```python
from build123d import *

# Parameters (mm, degrees)
SKETCH2_W            = 40
SKETCH2_H            = 40
SKETCH2_R            = 2.5
SKETCH2_R_2          = 16
SKETCH2_R_3          = 6.5
SKETCH2_R_4          = 12
BOSS_EXTRUDE5_DEPTH  = 2.5
BOSS_EXTRUDE8_START  = 2.5
SKETCH2_9_R          = 16
SKETCH2_9_R_2        = 6.5
SKETCH2_9_R_3        = 12
BOSS_EXTRUDE8_DEPTH  = 6
BOSS_EXTRUDE10_START = -32.5
SKETCH2_12_R         = 12
SKETCH2_12_R_2       = 6.5
BOSS_EXTRUDE10_DEPTH = 30
FILLET1_R            = 3
FILLET2_R            = 0.5
FILLET3_R            = 5
FILLET4_R            = 1


with BuildPart() as part:
    # Sketch2 → Boss-Extrude5 (new, symmetric)
    # profile 1 of 3: a face of its own
    with BuildSketch(Plane.XY):
        Rectangle(SKETCH2_W, SKETCH2_H)
        with Locations((-15, -15)):
            Circle(SKETCH2_R, mode=Mode.SUBTRACT)
        with Locations((15, -15)):
            Circle(SKETCH2_R, mode=Mode.SUBTRACT)
        with Locations((15, 15)):
            Circle(SKETCH2_R, mode=Mode.SUBTRACT)
        with Locations((-15, 15)):
            Circle(SKETCH2_R, mode=Mode.SUBTRACT)
        Circle(SKETCH2_R_2, mode=Mode.SUBTRACT)
    # profile 2 of 3: a face of its own
    with BuildSketch(Plane.XY):
        Circle(SKETCH2_R_2)
        Circle(SKETCH2_R_3, mode=Mode.SUBTRACT)
    # profile 3 of 3: a face of its own
    with BuildSketch(Plane.XY):
        Circle(SKETCH2_R_4)
        Circle(SKETCH2_R_3, mode=Mode.SUBTRACT)
    extrude(amount=BOSS_EXTRUDE5_DEPTH, both=True)

    # Sketch2<9> → Boss-Extrude8 (add)
    # profile 1 of 2: a face of its own
    with BuildSketch(Plane.XY.offset(BOSS_EXTRUDE8_START)):
        Circle(SKETCH2_9_R)
        Circle(SKETCH2_9_R_2, mode=Mode.SUBTRACT)
    # profile 2 of 2: a face of its own
    with BuildSketch(Plane.XY.offset(BOSS_EXTRUDE8_START)):
        Circle(SKETCH2_9_R_3)
        Circle(SKETCH2_9_R_2, mode=Mode.SUBTRACT)
    extrude(amount=BOSS_EXTRUDE8_DEPTH)

    # Sketch2<12> → Boss-Extrude10 (add)
    with BuildSketch(Plane.XY.offset(BOSS_EXTRUDE10_START)):
        Circle(SKETCH2_12_R)
        Circle(SKETCH2_12_R_2, mode=Mode.SUBTRACT)
    extrude(amount=BOSS_EXTRUDE10_DEPTH)

    # Fillet1
    fillet1_edges = [part.edges().sort_by_distance(p)[0] for p in [
        (20, -20, 0),
        (-20, -20, 0),
        (-20, 20, 0),
        (20, 20, 0),
    ]]
    fillet(fillet1_edges, radius=FILLET1_R)

    # Fillet2
    fillet2_edges = [part.edges().sort_by_distance(p)[0] for p in [
        (0, 20, -2.5),
        (20, 0, -2.5),
        (0, -20, -2.5),
        (-20, 0, -2.5),
        (-19.121320344, 19.121320344, -2.5),
        (-19.121320344, -19.121320344, -2.5),
        (19.121320344, -19.121320344, -2.5),
        (19.121320344, 19.121320344, -2.5),
    ]]
    fillet(fillet2_edges, radius=FILLET2_R)

    # Fillet3
    fillet3_edges = [part.edges().sort_by_distance(p)[0] for p in [
        (-12, 0, -2.5),
    ]]
    fillet(fillet3_edges, radius=FILLET3_R)

    # Fillet4
    fillet4_edges = [part.edges().sort_by_distance(p)[0] for p in [
        (-12, 0, -32.5),
    ]]
    fillet(fillet4_edges, radius=FILLET4_R)


solid = part.part
```
Geometry: final body of the model. Coordinates: model frame, mm. A direction names the side the tool comes from. Coordinates: 2 decimals unless noted, no trailing zeros. Order: outer loops, then holes, each group sorted by start corner. A loop starts at its lowest first (then second) coordinate and runs counter-clockwise, first axis right, second up. Notation, with made-up numbers: (9, -15) - (64, -15) arc R25 cw to (64, 18) - close; hole circle Ø10 at (72.25, 68). An arc over 180 degrees is marked (long way). Return JSON: item names as keys, results as strings. Group by question number.
1. Pin query (flat end, axial travel): pin 1 (6 mm diameter, centred on x = 15, y = 15, fed in from +Z); pin 2 (1 mm diameter, centred on y = -9.5, z = -9, fed in from -X); pin 3 (8 mm diameter, centred on x = 10.5, z = -13.5, fed in from +Y); pin 4 (5 mm diameter, centred on x = 15.5, z = -16, fed in from +Y). Return the tip coordinate at first contact, or that it passes through.
2. Set-up query: faces 4 (the face through (17, -4, -2.5)), 5 (the face through (0, 20, 0)). Return all of +Z, -Z, +X, -X, +Y, -Y with unobstructed straight access to the full face (end or side cutting, diameter ignored); none if empty.
3. Cut plane B-B (z = -11). Output: boundary loops of the cut face in (x, y), plus the area to 3 significant figures.
4. Cut plane A-A (x = 0). Output: boundary loops of the cut face in (y, z), plus the area to 3 significant figures.
5. Pull-direction query (X, two-part tool) for faces 1 (the face through (-9, 14, 2.5)), 2 (the face through (12.5, -14.9, 0)), 3 (the face through (-3.47, -15.62, 5.46)); classes: pulls with the +X half, pulls with the -X half, needs draft (parallel to the pull), parting line crosses it, or undercut.
6. Cut plane C-C (y = -15). Count the separate pieces of the cut face and the enclosed holes in it, plus the area to 3 significant figures.
7. Material intervals for line 1 along Y through (x, z) = (-15, -1); line 2 along Y through (x, z) = (0, -17.5); line 3 along X through (y, z) = (-6, -1), sorted ascending. Write a range as [from, to].
Resolved:
{
 "1": {"pin 1": "stops at z = 2.5", "pin 2": "stops at x = -7.94", "pin 3": "stops at y = 10.09", "pin 4": "passes through"},
 "2": {"face 4": "-Z", "face 5": "+Z, -Z, +X, -X, +Y"},
 "3": {"outline": "circle Ø24 at (0, 0); hole circle Ø13 at (0, 0)", "area": "320 mm²"},
 "4": {"outline": "(-20, -2) arc R0.5 ccw to (-19.5, -2.5) - (-17, -2.5) arc R5 cw to (-12, -7.5) - (-12, -31.5) arc R1 ccw to (-11, -32.5) - (-6.5, -32.5) - (-6.5, 8.5) - (-16, 8.5) - (-16, 2.5) - (-20, 2.5) - close; (6.5, -32.5) - (11, -32.5) arc R1 ccw to (12, -31.5) - (12, -7.5) arc R5 cw to (17, -2.5) - (19.5, -2.5) arc R0.5 ccw to (20, -2) - (20, 2.5) - (16, 2.5) - (16, 8.5) - (6.5, 8.5) - close", "area": "589 mm²"},
 "5": {"face 1": "needs draft", "face 2": "undercut", "face 3": "parting line crosses it"},
 "6": {"separate pieces": "3", "enclosed holes": "0", "area": "220 mm²"},
 "7": {"line 1": "y = [-20, -17.5], [-12.5, 12.5], [17.5, 20]", "line 2": "y = [-12, -6.5], [6.5, 12]", "line 3": "x = [-20, -2.5], [2.5, 20]"}
}
